Build history of the part. All positions in model axes, mm. A direction names the side the tool comes from. Give positions to 0.01 mm unless a question says otherwise; leave off trailing zeros. Write each loop counter-clockwise with the first axis right and the second up, starting at its lowest first coordinate (ties: lowest second). Pieces come first, ordered by that corner, then holes. Notation, with made-up numbers: M 60,-16.5 L 77,-16.5 A33 cw 77,15.5 Z; hole C 2.25,37.5 d1. An arc over 180 degrees is marked long. Return JSON: item names as keys, results as strings. Group by question number.
Q1. Wall check: probe 1 along Z at (x, y) = (-8, 1); probe 2 along Y at (x, z) = (-6.5, -5.75); probe 3 along X at (y, z) = (14, -3.5). Give the ranges that are in metal, low to high.
Q2. Flat gauge pins, fed straight in: pin 1 Ø5 at (y, z) = (13, -1) entering from -X; pin 2 Ø6 at (x, z) = (14.5, 0) entering from +Y; pin 3 Ø8 at (y, z) = (7, 0) entering from -X. Where does each tip first touch, or does it go through?
Q3. Band-saw the part on D-D, the plane z = 3.75. Give the cut face in (x, y), then the cut area to 3 significant figures.
Q4. Pull direction Y, two halves, no side cores. Call faces 5 (the flat face through (21.5, 15, -2)), 6 (the flat face through (0, 0, 2)), 7 (the flat face through (0, 2, 2)), 8 (the flat face through (21, 14, 1.5)): +Y half, -Y half, draft (parallel to the pull), parting line (faces both ways), or undercut.
Q5. Band-saw the part on C-C, the plane y = 18. Give the cut face in (x, z).
Q6. Band-saw the part on B-B, the plane x = -12. Give the cut face in (y, z).
Q7. Band-saw the part on A-A, the plane z = 0. Give the cut face in (x, y).
Q8. Tool access for faces 1 (the flat face through (20, 25, 0)), 2 (the flat face through (19.5, 14, -2)), 3 (the cylindrical face through (20.5, 5.5, 0)), 4 (the cylindrical face through (-15, 1, 0)): list every direction of +Z, -Z, +X, -X, +Y, -Y with a clear straight run to the whole face (end or side of a thin tool).
Autodesk Inventor part; units mm, degrees
ref_plane "YZ Plane" through (0, 0, 0) normal (1, 0, 0) x (0, 1, 0)
ref_plane "XZ Plane" through (0, 0, 0) normal (0, 1, 0) x (-1, 0, 0)
ref_plane "XY Plane" through (0, 0, 0) normal (0, 0, 1) x (1, 0, 0)
sketch "スケッチ1" plane through (0, 0, 0) normal (0, 1, 0) x (-1, 0, 0)
  line L0 (-17.5, 8) -> (17.5, 8)
  line L1 (17.5, 8) -> (17.5, -8)
  line L2 (17.5, -8) -> (-17.5, -8)
  line L3 (-17.5, -8) -> (-17.5, 8)
  line L4 (-17.5, 8) -> (17.5, -8) construction
  line L5 (17.5, 8) -> (-17.5, -8) construction
  point P0 (0, 0)
  dimension "d0" = 35
  dimension "d1" = 16
extrude "プレート1" add sketch "スケッチ1" along normal blind 2
sketch "スケッチ2" plane through (19.5, 4, -8) normal (1, 0, 0) x (0, 1, 0)
  line L0 (0, 16) -> (0, 0)
  line L1 (0, 0) -> (21, 0)
  line L2 (21, 0) -> (21, 16)
  line L3 (21, 16) -> (0, 16)
edge flange "フランジ1" height 25 angle 90 thickness 2 bend radius 2 thickness toward (1, 0, 0) relief tear relief width 2 relief depth 1 edges at (17.5, 2, 0) wall of the first edge with corners at (19.5, 4, 8) (19.5, 4, -8) (19.5, 25, -8) (19.5, 25, 8)
bend "曲げ1"
corner "コーナー1"
sketch "スケッチ3" plane through (21.5, 25, 8) normal (1, 0, 0) x (0, 0, -1)
  line L0 (6.5, -4) -> (6.5, -18)
  arc A0 (6.5, -18) -> (9.5, -18) centre (8, -18) ccw
  line L1 (9.5, -18) -> (9.5, -4)
  arc A1 (9.5, -4) -> (6.5, -4) centre (8, -4) ccw
  line L2 (16, 0) -> (16, -21)
  line L3 (0, 0) -> (16, 0)
  point P0 (8, -25)
  point P1 (8, 0)
  dimension "d19" = 1.5
extrude "押し出し1" cut sketch "スケッチ3" against normal blind 10
sketch "スケッチ4" plane through (0, 2, 0) normal (0, 1, 0) x (1, 0, 0)
  line L0 (-13.5, -1.5) -> (13.5, -1.5)
  arc A0 (13.5, -1.5) -> (13.5, 1.5) centre (13.5, 0) ccw
  line L1 (13.5, 1.5) -> (-13.5, 1.5)
  arc A1 (-13.5, 1.5) -> (-13.5, -1.5) centre (-13.5, 0) ccw
  line L2 (-17.5, -8) -> (-17.5, 8)
  line L3 (17.5, 8) -> (17.5, -8)
  point P0 (0, 0)
  dimension "d23" = 4
  dimension "d24" = 4
  dimension "d25" = 1.5
extrude "押し出し2" cut sketch "スケッチ4" against normal blind 10
equation "\"d2\" = Thickness"
equation "\"d3\" = BendReliefWidth"
equation "\"d4\" = BendReliefDepth"
equation "\"d5\" = MinimumRemnant"
equation "\"d6\" = TransitionRadius"
equation "\"d9\" = BendRadius"
equation "\"d10\" = CornerReliefSize"
equation "\"d11\" = GapSize"
equation "\"d12\" = JacobiRadiusSize"
equation "\"BendRadius\" = Thickness"
equation "\"BendReliefWidth\" = Thickness"
equation "\"BendReliefDepth\" = 0.5 * Thickness"
equation "\"CornerReliefSize\" = 4 * Thickness"
equation "\"MinimumRemnant\" = 2 * Thickness"
equation "\"TransitionRadius\" = BendRadius"
equation "\"JacobiRadiusSize\" = BendRadius"
equation "\"GapSize\" = Thickness"
properties part number "keyL_extended" material "アルミニウム 6061"
From the geometry:
{
 "1": {"probe 1": "z = -8 to -1.5, 1.5 to 8", "probe 2": "y = 0 to 2", "probe 3": "x = 19.5 to 21.5"},
 "2": {"pin 1": "stops at x = 19.5", "pin 2": "stops at y = 2", "pin 3": "stops at x = 19.23"},
 "3": {"outline": "M -17.5,0 L 17.5,0 A4 ccw 21.5,4 L 21.5,25 L 19.5,25 L 19.5,4 A2 cw 17.5,2 L -17.5,2 Z", "area": "121 mm^2"},
 "4": {"face 5": "draft", "face 6": "-Y half", "face 7": "+Y half", "face 8": "undercut"},
 "5": {"outline": "M 19.5,-8 L 21.5,-8 L 21.5,-1.5 L 19.5,-1.5 Z; M 19.5,1.5 L 21.5,1.5 L 21.5,8 L 19.5,8 Z"},
 "6": {"outline": "M 0,-8 L 2,-8 L 2,-1.5 L 0,-1.5 Z; M 0,1.5 L 2,1.5 L 2,8 L 0,8 Z"},
 "7": {"outline": "M -17.5,0 L -15,0 L -15,2 L -17.5,2 Z; M 15,0 L 17.5,0 A4 ccw 21.5,4 L 21.5,5.5 L 19.5,5.5 L 19.5,4 A2 cw 17.5,2 L 15,2 Z; M 19.5,22.5 L 21.5,22.5 L 21.5,25 L 19.5,25 Z"},
 "8": {"face 1": "+Z, -Z, +X, -X, +Y", "face 2": "+Z, -Z, -X, +Y", "face 3": "+X, -X", "face 4": "+Y, -Y"}
}
